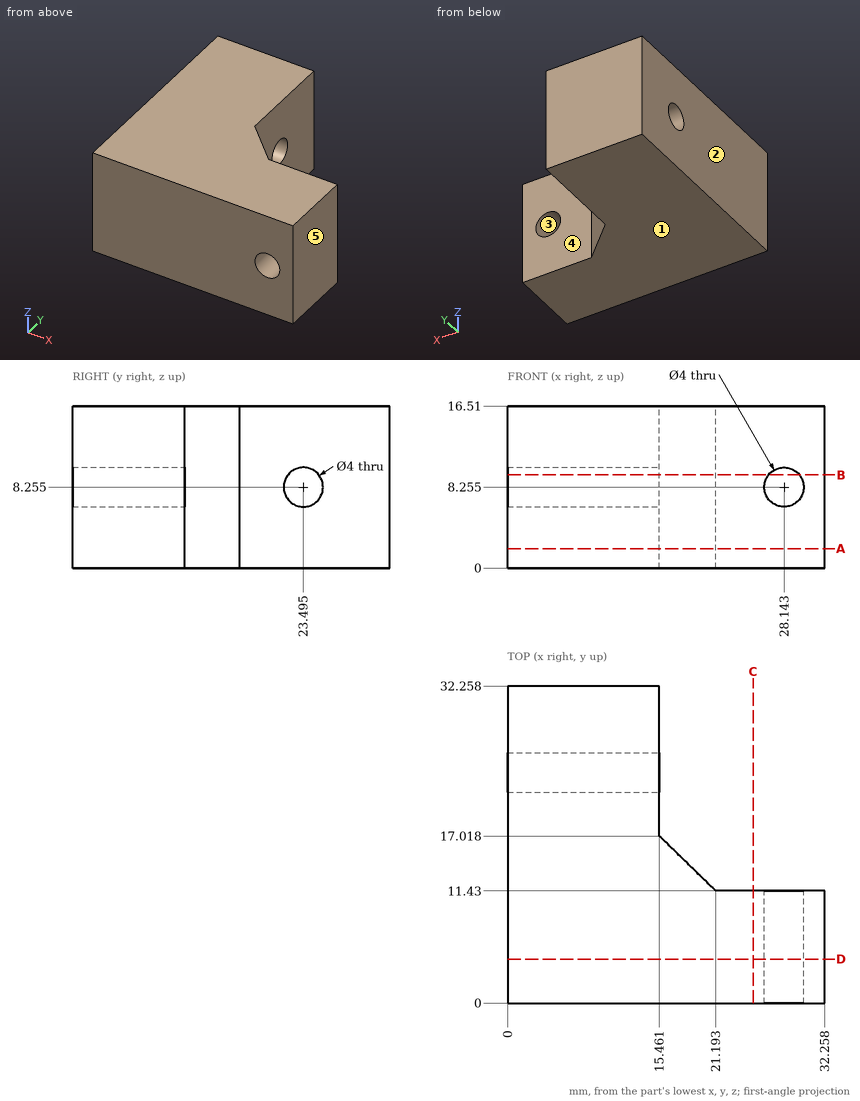
Part print with two shaded views. Sizes in mm from the minimum x, y, z corner. A direction names the side the tool comes from. Coordinates: 2 decimals unless noted, no trailing zeros. Write each loop counter-clockwise with the first axis right and the second up, starting at its lowest first coordinate (ties: lowest second). Pieces come first, ordered by that corner, then holes. Notation, with made-up numbers: (-20, 85) - (14, 85) arc R16 cw to (14, 93) - close; hole circle Ø1 at (45, 64). An arc over 180 degrees is marked (long way). Use a Markdown table: item, result. Add a question column.
Item 1: Drop a flat-ended pin along its axis: pin 1 (3.5 mm diameter, centred on x = 25, z = 9, fed in from +Y). Give the stop position or say it passes through.
Item 2: Band-saw the part on A-A, the plane z = 2. Write the cut outline in (x, y), and give its area (3 significant figures).
Item 3: Drill centre lines: line 1 along X through (y, z) = (21, 2.5); line 2 along X through (y, z) = (6, 6.75) (1 decimal); line 3 along Y through (x, z) = (3, 8.75). Where is each one in solid material? Low to high.
Item 4: Band-saw the part on C-C, the plane x = 25. Write the cut outline in (y, z).
Item 5: Band-saw the part on D-D, the plane y = 4.5. Write the cut outline in (x, z) (1 decimal).
Item 6: Two-plate mould, pull along X, no slides. Class the marked faces 1, 2 and 3: pulls with the +X half, pulls with the -X half, needs draft (parallel to the pull), parting line crosses it, or undercut.
Item 7: Band-saw the part on B-B, the plane z = 9.5. Write the cut outline in (x, y).
Item 8: 3-axis set-ups, long thin cutter, end or side, ignore diameter. For the marked faces 4 and 5: which of +Z, -Z, +X, -X, +Y, -Y reach the whole face in a straight line?
A:
| question | item | result |
|---|---|---|
| 1 | pin 1 | stops at y = 11.43 |
| 2 | outline | (0, 0) - (32.26, 0) - (32.26, 11.43) - (21.19, 11.43) - (15.46, 17.02) - (15.46, 32.26) - (0, 32.26) - close |
| 2 | area | 707 mm² |
| 3 | line 1 | x = 0 to 15.46 |
| 3 | line 2 | x = 0 to 26.8, 29.5 to 32.3 |
| 3 | line 3 | y = 0 to 21.56, 25.43 to 32.26 |
| 4 | outline | (0, 0) - (11.43, 0) - (11.43, 16.51) - (0, 16.51) - close |
| 5 | outline | (0, 0) - (32.3, 0) - (32.3, 16.5) - (0, 16.5) - close; hole circle Ø4 at (28.1, 8.3) |
| 6 | face 1 | needs draft |
| 6 | face 2 | pulls with the -X half |
| 6 | face 3 | undercut |
| 7 | outline | (0, 0) - (26.58, 0) - (26.58, 11.43) - (21.19, 11.43) - (15.46, 17.02) - (15.46, 21.93) - (0, 21.93) - close; (0, 25.06) - (15.46, 25.06) - (15.46, 32.26) - (0, 32.26) - close; (29.71, 0) - (32.26, 0) - (32.26, 11.43) - (29.71, 11.43) - close |
| 8 | face 4 | +Z, -Z, +X, +Y |
| 8 | face 5 | +Z, -Z, +X, +Y, -Y |
